from build123d import *

# Parameters (mm, degrees)
SKETCH1_W           = 307
SKETCH1_H           = 230
BOSS_EXTRUDE1_DEPTH = 160
BOSS_EXTRUDE2_START = 80
SKETCH1_3_W         = 23
SKETCH1_3_H         = 230
BOSS_EXTRUDE2_DEPTH = 5


with BuildPart() as part:
    # Sketch1 → Boss-Extrude1 (new body)
    with BuildSketch(Plane(origin=(0, 0, 0), x_dir=(1, 0, 0), z_dir=(0, 1, 0))):
        Rectangle(SKETCH1_W, SKETCH1_H)
    extrude(amount=BOSS_EXTRUDE1_DEPTH)

    # Sketch1<3> → Boss-Extrude2 (add)
    with BuildSketch(Plane(origin=(0, 0, 0), x_dir=(1, 0, 0), z_dir=(0, 1, 0)).offset(BOSS_EXTRUDE2_START)):
        with Locations((-165, 0)):
            Rectangle(SKETCH1_3_W, SKETCH1_3_H)
        with Locations((165, 0)):
            Rectangle(SKETCH1_3_W, SKETCH1_3_H)
    extrude(amount=BOSS_EXTRUDE2_DEPTH)


solid = part.part
The listing builds one solid part. Answer for the finished solid, in the listing's coordinates (mm). A direction names the side the tool comes from. Round coordinates to 2 decimals unless told otherwise and drop trailing zeros. Order: outer loops, then holes, each group sorted by start corner. A loop starts at its lowest first (then second) coordinate and runs counter-clockwise, first axis right, second up. Notation, with made-up numbers: (-8.75, -26.75) -> (-3.75, -26.75) arc R28 ccw to (-3.75, -5.75) -> close; hole circle Ø4 at (-39.75, -36). An arc over 180 degrees is marked (long way). Put each result on its own line as item: value.
Q1. Section B-B, the plane y = 58 is taken. Write down the section's boundary in (x, z), and give its area (3 significant figures).
Results list:
outline: (-153.5, -115) -> (153.5, -115) -> (153.5, 115) -> (-153.5, 115) -> close
area: 70,600 mm^2
Q2. Each of these flat-tipped pins is pushed along its axis until it touches: P1, Ø22.5, axis at y = 116.5, z = -4, coming from the -X side; P2, Ø11.5, axis at x = 169, z = 17, coming from the -Y side; P3, Ø18.5, axis at x = 166.5, z = -25.5, coming from the +Y side. Where does it stop, or does it pass through?
Results list:
P1: x = -153.5
P2: y = 80
P3: y = 85
Q3. Which of the six approach directions +Z, -Z, +X, -X, +Y, -Y give full straight-line access (tool end or side, diameter ignored) to faces 1 (the flat face through (153.5, 122, 2)), 2 (the flat face through (-165, 80, -2)), 3 (the flat face through (153.5, 39, 2))?
Results list:
face 1: +Z, -Z, +X, +Y
face 2: +Z, -Z, -X, -Y
face 3: +Z, -Z, +X, -Y
Q4. Section A-A, the plane z = -25 is taken. Write down the section's boundary in (x, y), and give its area (4 significant figures).
Results list:
outline: (-176.5, 80) -> (-153.5, 80) -> (-153.5, 0) -> (153.5, 0) -> (153.5, 80) -> (176.5, 80) -> (176.5, 85) -> (153.5, 85) -> (153.5, 160) -> (-153.5, 160) -> (-153.5, 85) -> (-176.5, 85) -> close
area: 49,350 mm^2
Q5. Consider line 1 along X through (y, z) = (49.5, 13); line 2 along Y through (x, z) = (155, -2). Determine where each line is inside the solid, lowest interval first.
Results list:
line 1: -153.5 to 153.5
line 2: 80 to 85
